Can you work these out from the drawing? Everything is in mm from the part's minimum corner. Give positions to 0.01 mm unless a question says otherwise; leave off trailing zeros. Write each loop counter-clockwise with the first axis right and the second up, starting at its lowest first coordinate (ties: lowest second). Pieces come first, ordered by that corner, then holes. Notation, with made-up numbers: M -24.5,-27.5 L -17.5,-27.5 A38 cw -17.5,10.5 Z; hole C 11,56 d3. An arc over 180 degrees is marked long. One line per item, written item: value.
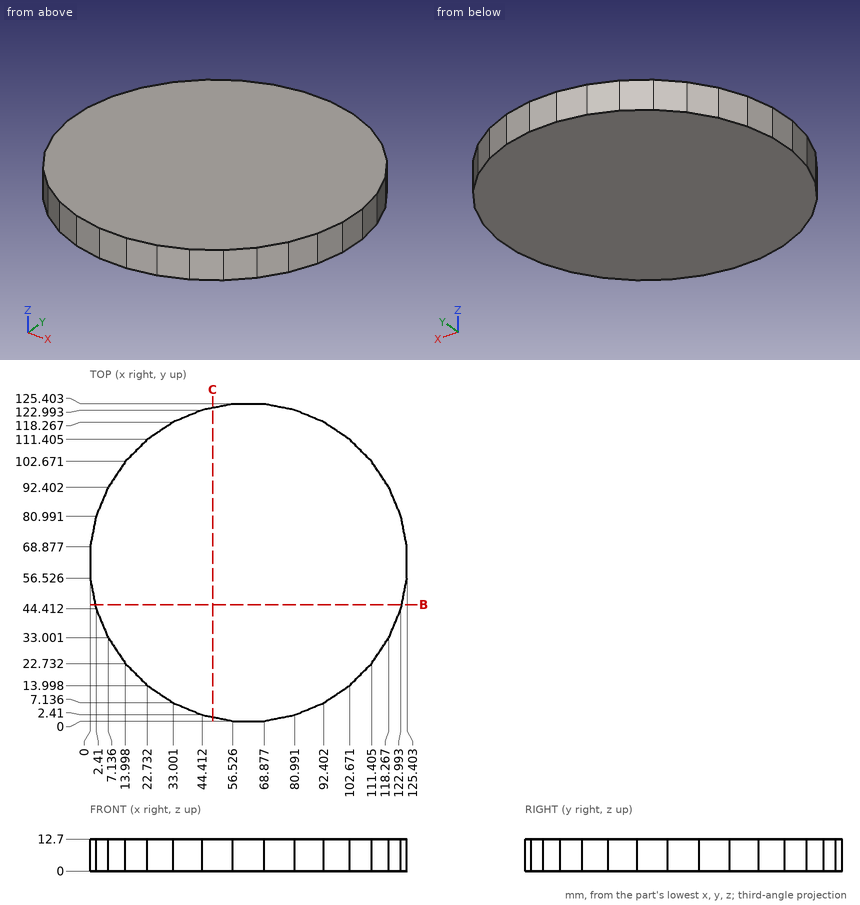
1) If we section it at C-C, the plane x = 48.5: Write out the boundary of the cut face in (y, z).
Outcome:
outline: M 1.6,0 L 123.81,0 L 123.81,12.7 L 1.6,12.7 Z
2) Please list where these lines run through material, in increasing order: L1, parallel to X at y = 33, z = 2 (1 decimal); L2, parallel to Y at x = 56.5, z = 2 (1 decimal); L3, parallel to X at y = 51, z = 5.5. Write a range as from..to.
Outcome:
L1: x = 7.1..118.3
L2: y = 0..125.4
L3: x = 1.1..124.3
3) If we section it at B-B, the plane y = 46: Write out the boundary of the cut face in (x, z), then the cut area to 3 significant figures.
Outcome:
outline: M 2.09,0 L 123.31,0 L 123.31,12.7 L 2.09,12.7 Z
area: 1,540 mm^2
4) I'm going to push flat-ended pins straight in: pin 1 (6 mm diameter, centred on y = 89.5, z = 7, fed in from -X); pin 2 (2 mm diameter, centred on x = 72, z = 7.5, fed in from -Y); pin 3 (2 mm diameter, centred on x = 55, z = 8.5, fed in from -Y) (1 decimal). Where does each tip first touch, or does it pass through?
Outcome:
pin 1: stops at x = 4.69
pin 2: stops at y = 0.42
pin 3: stops at y = 0.1
